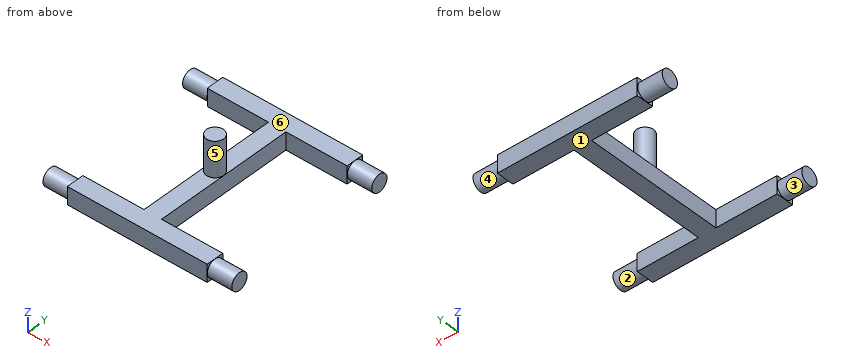
from build123d import *

# Parameters (mm, degrees)
CROQUIS2_W               = 400
CROQUIS2_H               = 500
SALIENTE_EXTRUIR3_DEPTH  = 50
CROQUIS7_W               = 175
CROQUIS7_H               = 400
CORTAR_EXTRUIR2_DEPTH    = 50
CROQUIS9_R               = 24.5
SALIENTE_EXTRUIR5_DEPTH  = 70
CROQUIS10_R              = 24.5
SALIENTE_EXTRUIR6_DEPTH  = 70
CROQUIS19_R              = 24.5
SALIENTE_EXTRUIR10_DEPTH = 70
CROQUIS20_R              = 24.5
SALIENTE_EXTRUIR11_DEPTH = 70
CROQUIS12_R              = 24.5
SALIENTE_EXTRUIR12_DEPTH = 100


with BuildPart() as part:
    # Croquis2 → Saliente-Extruir3 (new body)
    with BuildSketch(Plane.XY):
        Rectangle(CROQUIS2_W, CROQUIS2_H)
    extrude(amount=-SALIENTE_EXTRUIR3_DEPTH)

    # Croquis7 → Cortar-Extruir2 (cut)
    with BuildSketch(Plane.XY):
        with Locations((-112.5, 0)):
            Rectangle(CROQUIS7_W, CROQUIS7_H)
        with Locations((112.5, 0)):
            Rectangle(CROQUIS7_W, CROQUIS7_H)
    extrude(amount=-CORTAR_EXTRUIR2_DEPTH, mode=Mode.SUBTRACT)

    # Croquis9 → Saliente-Extruir5 (add)
    with BuildSketch(Plane.ZY.offset(200)):
        with Locations((-25, -225.045105614)):
            Circle(CROQUIS9_R)
    extrude(amount=SALIENTE_EXTRUIR5_DEPTH)

    # Croquis10 → Saliente-Extruir6 (add)
    with BuildSketch(Plane.ZY.offset(200)):
        with Locations(Location((-25, 223.724834231, 0), (0, 0, 255.54880869))):
            Circle(CROQUIS10_R)
    extrude(amount=SALIENTE_EXTRUIR6_DEPTH)

    # Croquis19 → Saliente-Extruir10 (add)
    with BuildSketch(Plane(origin=(200, 0, 0), x_dir=(0, 0, -1), z_dir=(1, 0, 0))):
        with Locations((25, -225)):
            Circle(CROQUIS19_R)
    extrude(amount=SALIENTE_EXTRUIR10_DEPTH)

    # Croquis20 → Saliente-Extruir11 (add)
    with BuildSketch(Plane(origin=(200, 0, 0), x_dir=(0, 0, -1), z_dir=(1, 0, 0))):
        with Locations((25, 225)):
            Circle(CROQUIS20_R)
    extrude(amount=SALIENTE_EXTRUIR11_DEPTH)

    # Croquis12 → Saliente-Extruir12 (add)
    with BuildSketch(Plane.XY):
        with Locations(Location((0, 0, 0), (0, 0, 180))):
            Circle(CROQUIS12_R)
    extrude(amount=SALIENTE_EXTRUIR12_DEPTH)


solid = part.part
For this review, take the finished solid that the model builds, in its own axes (mm). Face numbers are marked on the shaded views. A direction names the side the tool comes from. Coordinates: 2 decimals unless noted, no trailing zeros. Loops run counter-clockwise (first coordinate to the right, second up) from the corner with the lowest first, then second, coordinate; pieces in that order, holes last. Notation, with made-up numbers: (44.25, 84) -> (90.25, 84) arc R16 ccw to (90.25, 105) -> close; hole circle Ø6 at (30, -34.5). An arc over 180 degrees is marked (long way). Write each question's results on one line, items separated by ' | '.
Q1. Add section C-C, the plane z = -25. State the section outline as (x, y) points, then the cut area to 3 significant figures.
Taken from the geometry:
outline: (-270, -249.55) -> (-200, -249.55) -> (-200, -250) -> (200, -250) -> (200, -249.5) -> (270, -249.5) -> (270, -200.5) -> (200, -200.5) -> (200, -200) -> (25, -200) -> (25, 200) -> (200, 200) -> (200, 200.5) -> (270, 200.5) -> (270, 249.5) -> (200, 249.5) -> (200, 250) -> (-200, 250) -> (-200, 248.22) -> (-270, 248.22) -> (-270, 199.22) -> (-200, 199.22) -> (-200, 200) -> (-25, 200) -> (-25, -200) -> (-200, -200) -> (-200, -200.55) -> (-270, -200.55) -> close | area: 73,700 mm²
Q2. Mouldability with a two-part tool opening along Y and no side actions: class the marked faces 4, 5 and 6 as +Y half, -Y half, draft (parallel to the pull), parting line (faces both ways), or undercut.
Taken from the geometry:
face 4: undercut | face 5: parting line | face 6: draft
Q3. Add section A-A, the plane x = 75.5. State the section outline as (y, z) points, then the cut area to 3 significant figures.
Taken from the geometry:
outline: (-250, -50) -> (-200, -50) -> (-200, 0) -> (-250, 0) -> close; (200, -50) -> (250, -50) -> (250, 0) -> (200, 0) -> close | area: 5,000 mm²
Q4. Add section D-D, the plane x = 0. State the section outline as (y, z) points.
Taken from the geometry:
outline: (-250, -50) -> (250, -50) -> (250, 0) -> (24.5, 0) -> (24.5, 100) -> (-24.5, 100) -> (-24.5, 0) -> (-250, 0) -> close
Q5. For pin 1 Ø0.6 at (y, z) = (199.5, -27) entering from +X; pin 2 Ø12 at (x, y) = (35, 55.5) entering from +Z; pin 3 Ø15 at (y, z) = (86, -15) entering from -X, all flat-tipped, find the tip position at first contact; note any pin that passes through.
Taken from the geometry:
pin 1: x = 25 | pin 2: through | pin 3: x = -25
Q6. To check wall thickness, follow line 1 along Y through (x, z) = (65, -28); line 2 along Z through (x, y) = (104, 204); line 3 along Y through (x, z) = (-237, -32). State the ranges of each line that lie inside material, in increasing order. Write a range as [from, to].
Taken from the geometry:
line 1: [-250, -200], [200, 250] | line 2: [-50, 0] | line 3: [-248.52, -201.57], [200.25, 247.2]
Q7. Machinability: for the marked faces 1, 2 and 3, which of the approach directions +Z, -Z, +X, -X, +Y, -Y give a long, thin tool a straight path to every point of the face, cutting with its end or side? Answer none if there is none.
Taken from the geometry:
face 1: -Z, +X, -X, +Y, -Y | face 2: +X | face 3: -X
Q8. Add section B-B, the plane y = 0. State the section outline as (x, z) points, then the cut area to 3 significant figures.
Taken from the geometry:
outline: (-25, -50) -> (25, -50) -> (25, 0) -> (24.5, 0) -> (24.5, 100) -> (-24.5, 100) -> (-24.5, 0) -> (-25, 0) -> close | area: 7,400 mm²
